Part print with two shaded views. Sizes in mm from the minimum x, y, z corner. A direction names the side the tool comes from. Round coordinates to 2 decimals unless told otherwise and drop trailing zeros. Loops run counter-clockwise (first coordinate to the right, second up) from the corner with the lowest first, then second, coordinate; pieces in that order, holes last. Notation, with made-up numbers: (76, 80.5) - (113, 80.5) arc R16 ccw to (113, 100.5) - close; hole circle Ø11 at (15, 34). An arc over 180 degrees is marked (long way). One line per question, with ' | ' between items.
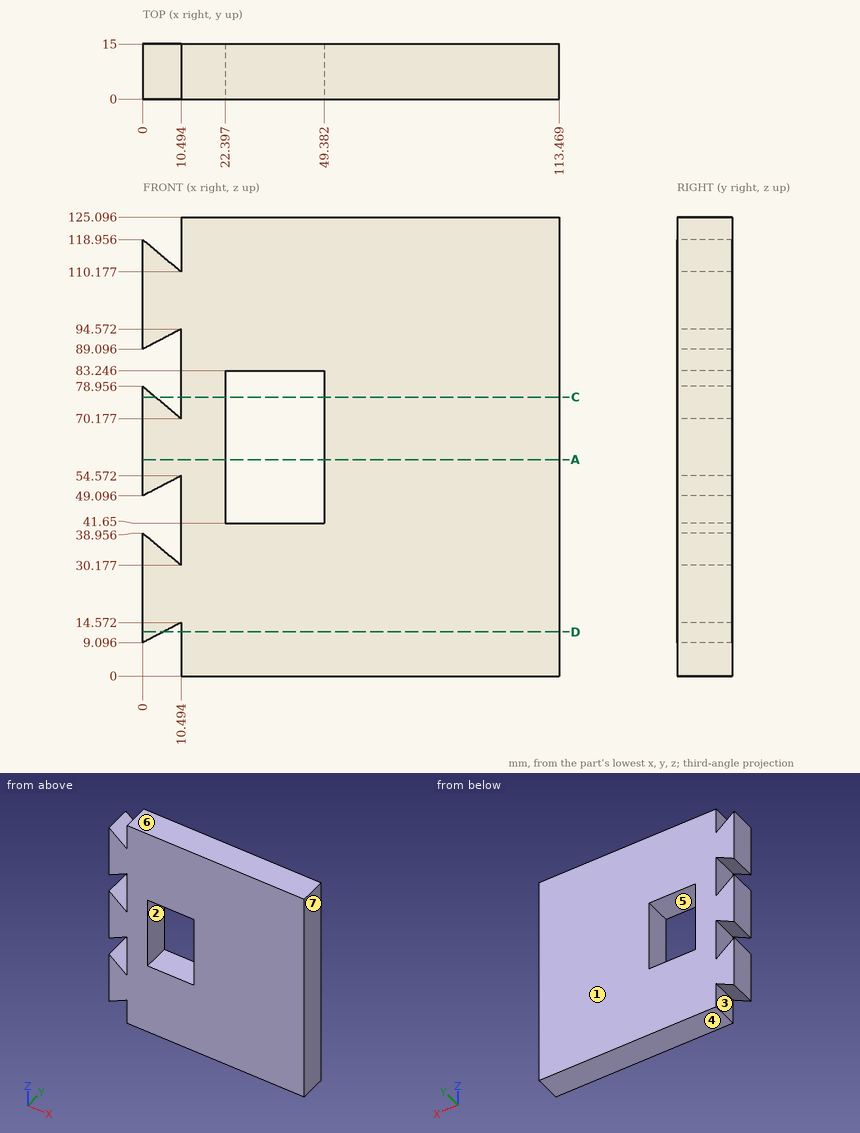
(1) Cut at C-C, the plane z = 76. Write the cut outline in (x, y) (1 decimal).
Results found:
outline: (0, 0) - (3.5, 0) - (3.5, 15) - (0, 15) - close; (10.5, 0) - (22.4, 0) - (22.4, 15) - (10.5, 15) - close; (49.4, 0) - (113.5, 0) - (113.5, 15) - (49.4, 15) - close
(2) Drop a flat-ended pin along its axis: P1, Ø2, axis at y = 8, z = 88, coming from the -X side. Give the stop position or say it passes through.
Results found:
P1: stops at x = 10.49
(3) Two-plate mould, pull along Z, no slides. Class the marked faces 4, 5, 6 and 7: released by +Z, released by -Z, zero draft, split by the parting line, or undercut.
Results found:
face 4: released by -Z | face 5: undercut | face 6: released by +Z | face 7: zero draft
(4) Probe L1, parallel to X at y = 3.75, z = 73.5 (1 decimal); L2, parallel to X at y = 13, z = 63.5; L3, parallel to X at y = 4.5, z = 9 (1 decimal). List the from-to ranges inside material, lowest first.
Results found:
L1: x = 0 to 6.5, 10.5 to 22.4, 49.4 to 113.5 | L2: x = 0 to 22.4, 49.38 to 113.47 | L3: x = 10.5 to 113.5
(5) Tool access for the marked faces 1, 2 and 3: list every direction of +Z, -Z, +X, -X, +Y, -Y with a clear straight run to the whole face (end or side of a thin tool).
Results found:
face 1: +Z, -Z, +X, -X, +Y | face 2: +Y, -Y | face 3: -Z, +Y, -Y
(6) Cut at A-A, the plane z = 59. Write the cut outline in (x, y).
Results found:
outline: (0, 0) - (22.4, 0) - (22.4, 15) - (0, 15) - close; (49.38, 0) - (113.47, 0) - (113.47, 15) - (49.38, 15) - close
(7) Cut at D-D, the plane z = 12. Write the cut outline in (x, y) (1 decimal).
Results found:
outline: (0, 0) - (5.6, 0) - (5.6, 15) - (0, 15) - close; (10.5, 0) - (113.5, 0) - (113.5, 15) - (10.5, 15) - close
